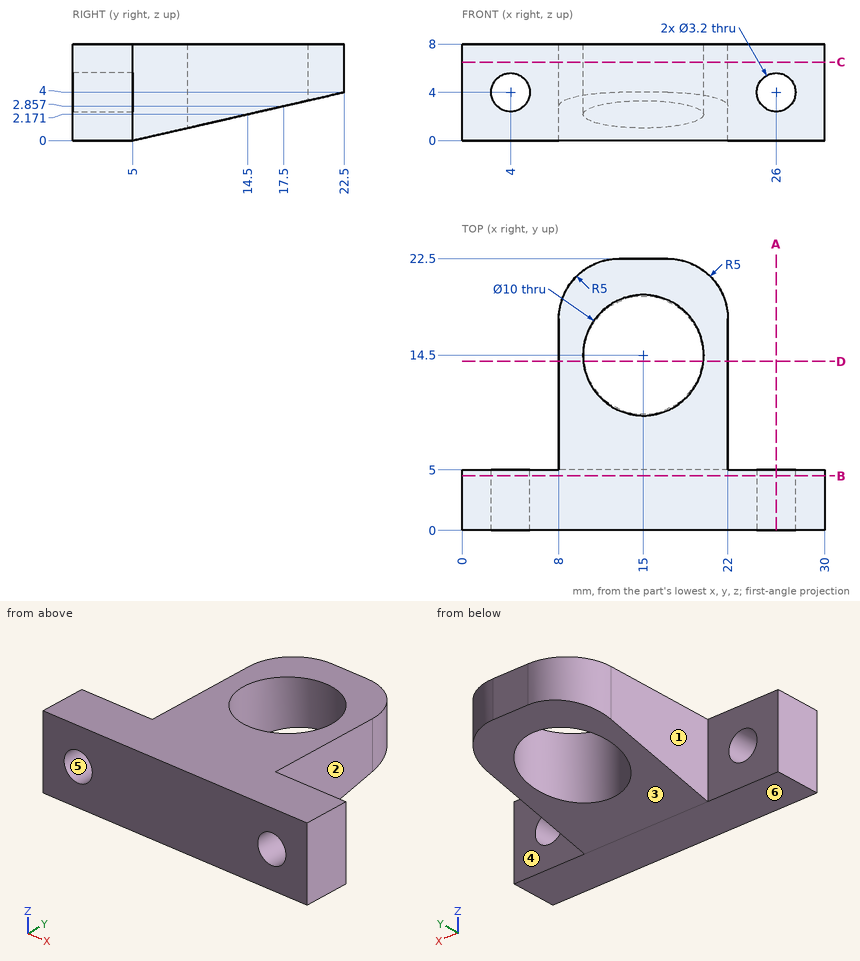
Drawing for the job (mm, zero at the part's lowest x, y, z). A direction names the side the tool comes from. Round coordinates to 2 decimals unless told otherwise and drop trailing zeros. Order: outer loops, then holes, each group sorted by start corner. A loop starts at its lowest first (then second) coordinate and runs counter-clockwise, first axis right, second up. Notation, with made-up numbers: M -23.5,78.25 L 6.5,78.25 A26 ccw 6.5,93.25 Z; hole C 51.25,10 d6. An arc over 180 degrees is marked long. Use one line per item in the form item = value.
Q1. Which spindle directions (+Z, -Z, +X, -X, +Y, -Y) get a long thin tool onto all of the face, cutting with end or side? Do the marked faces 1, 2 and 3. Say none if no direction does.
Recorded:
face_1 = +Z, -Z, -X, +Y
face_2 = +Z, -Z, +X, +Y
face_3 = -Z, +X, -X, +Y
Q2. Two-plate mould, pull along Z, no slides. Class the marked faces 4, 5 and 6: +Z half, -Z half, draft (parallel to the pull), parting line (faces both ways), or undercut.
Recorded:
face_4 = draft
face_5 = undercut
face_6 = -Z half
Q3. Probe L1, parallel to X at y = 14.5, z = 5.5; L2, parallel to Y at x = 15, z = 6; L3, parallel to Z at x = 26, y = 1.3. List the from-to ranges inside material, lowest first.
Recorded:
L1 = 8 to 10, 20 to 22
L2 = 0 to 9.5, 19.5 to 22.5
L3 = 0 to 2.4, 5.6 to 8
Q4. Saw through at C-C on z = 6.5. Give the cut face in (x, y), then the cut area to 3 significant figures.
Recorded:
outline = M 0,0 L 30,0 L 30,5 L 22,5 L 22,17.5 A5 ccw 17,22.5 L 13,22.5 A5 ccw 8,17.5 L 8,5 L 0,5 Z; hole C 15,14.5 d10
area = 306 mm^2
Q5. Saw through at B-B on y = 4.5. Give the cut face in (x, z).
Recorded:
outline = M 0,0 L 30,0 L 30,8 L 0,8 Z; hole C 4,4 d3.2; hole C 26,4 d3.2
Q6. Flat gauge pins, fed straight in: P1, Ø1.5, axis at y = 9, z = 6.5, coming from the +X side; P2, Ø4, axis at x = 28, z = 5.5, coming from the +Y side; P3, Ø2.5, axis at x = 26, z = 4, coming from the +Y side (3 decimals). Where does each tip first touch, or does it go through?
Recorded:
P1 = 22
P2 = 5
P3 = through
Q7. Saw through at D-D on y = 14. Give the cut face in (x, z) (1 decimal).
Recorded:
outline = M 8,2.1 L 10,2.1 L 10,8 L 8,8 Z; M 20,2.1 L 22,2.1 L 22,8 L 20,8 Z
Q8. Saw through at A-A on x = 26. Give the cut face in (y, z), then the cut area to 3 significant figures.
Recorded:
outline = M 0,0 L 5,0 L 5,2.4 L 0,2.4 Z; M 0,5.6 L 5,5.6 L 5,8 L 0,8 Z
area = 24.0 mm^2
